Verification items for this drawing (mm, ordinates from the low corner). A direction names the side the tool comes from. Coordinates: 2 decimals unless noted, no trailing zeros. Write each loop counter-clockwise with the first axis right and the second up, starting at its lowest first coordinate (ties: lowest second). Pieces come first, ordered by that corner, then holes. Notation, with made-up numbers: (20, 45) -> (26, 45) arc R13 ccw to (26, 56) -> close; hole circle Ø8 at (23, -2). An arc over 180 degrees is marked (long way). One line per question, with ' | ' between items.
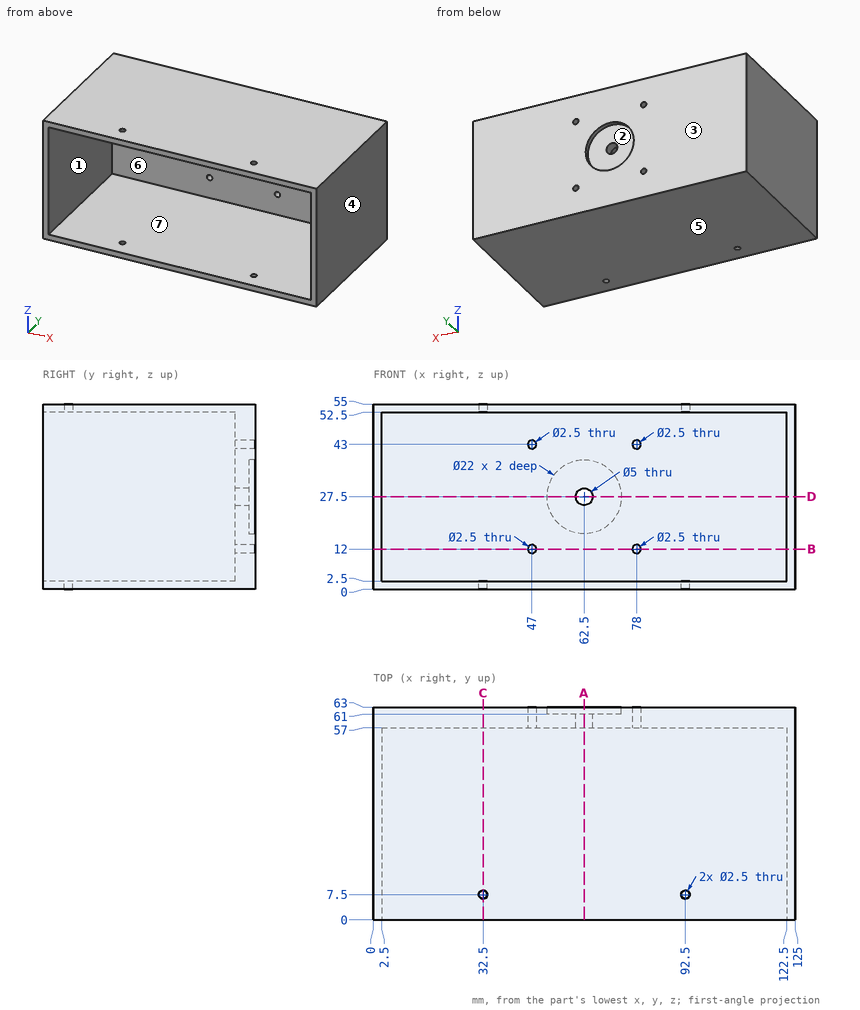
(1) Material ranges on line 1 (Z direction, x = 47, y = 58); line 2 (X direction, y = 58.8, z = 43); line 3 (Z direction, x = 15, y = 46), recorded low to high.
Answers below:
line 1: z = 0 to 10.75, 13.25 to 41.75, 44.25 to 55 | line 2: x = 0 to 45.75, 48.25 to 76.75, 79.25 to 125 | line 3: z = 0 to 2.5, 52.5 to 55
(2) Cross-section at C-C (x = 32.5). Record the cut outline in (y, z), plus the area to 4 significant figures.
Answers below:
outline: (0, 0) -> (6.25, 0) -> (6.25, 2.5) -> (0, 2.5) -> close; (0, 52.5) -> (6.25, 52.5) -> (6.25, 55) -> (0, 55) -> close; (8.75, 0) -> (63, 0) -> (63, 55) -> (8.75, 55) -> (8.75, 52.5) -> (57, 52.5) -> (57, 2.5) -> (8.75, 2.5) -> close | area: 602.5 mm²
(3) Cross-section at B-B (z = 12). Record the cut outline in (x, y), plus the area to 4 significant figures.
Answers below:
outline: (0, 0) -> (2.5, 0) -> (2.5, 57) -> (45.75, 57) -> (45.75, 63) -> (0, 63) -> close; (48.25, 57) -> (76.75, 57) -> (76.75, 63) -> (48.25, 63) -> close; (79.25, 57) -> (122.5, 57) -> (122.5, 0) -> (125, 0) -> (125, 63) -> (79.25, 63) -> close | area: 1,005 mm²
(4) Tool access check on the marked faces 1, 2 and 3. Record the directions out of +Z, -Z, +X, -X, +Y, -Y that give a thin tool (end or side, any length) a straight path to the whole face; none if there is none.
Answers below:
face 1: -Y | face 2: +Y | face 3: +Z, -Z, +X, -X, +Y
(5) Draft check along Z on the marked faces 4, 5, 6 and 7. Enter one of: pulls with the +Z half, pulls with the -Z half, needs draft (parallel to the pull), parting line crosses it, or undercut.
Answers below:
face 4: needs draft | face 5: pulls with the -Z half | face 6: undercut | face 7: undercut
(6) Cross-section at A-A (x = 62.5). Record the cut outline in (y, z), plus the area to 3 significant figures.
Answers below:
outline: (0, 0) -> (63, 0) -> (63, 16.5) -> (61, 16.5) -> (61, 25) -> (57, 25) -> (57, 2.5) -> (0, 2.5) -> close; (0, 52.5) -> (57, 52.5) -> (57, 30) -> (61, 30) -> (61, 38.5) -> (63, 38.5) -> (63, 55) -> (0, 55) -> close | area: 551 mm²
(7) Depth check by flat-ended pin: P1, Ø3, axis at x = 78, z = 12, coming from the -Y side; P2, Ø11, axis at x = 63, z = 24.5, coming from the +Y side. Enter the tip coordinate at first touch or a pass-through.
Answers below:
P1: stops at y = 57 | P2: stops at y = 61
(8) Cross-section at D-D (z = 27.5). Record the cut outline in (x, y).
Answers below:
outline: (0, 0) -> (2.5, 0) -> (2.5, 57) -> (60, 57) -> (60, 61) -> (51.5, 61) -> (51.5, 63) -> (0, 63) -> close; (65, 57) -> (122.5, 57) -> (122.5, 0) -> (125, 0) -> (125, 63) -> (73.5, 63) -> (73.5, 61) -> (65, 61) -> close
